from build123d import *

# Parameters (mm, degrees)
F2_R     = 19.05
F3_DEPTH = 55.881
F4_R     = 3.048
F5_R     = 6.35
F6_DEPTH = 19.051


with BuildPart() as f1:
    # F0 (on Front) → F1 (revolve)
    with BuildSketch(Plane.XZ):
        Polygon((0, 55.88), (0, 0), (69.85, 0), (69.85, 19.05), (35.052, 19.05), (35.052, 55.88), align=None)
    revolve(axis=Axis((0, 0, 27.94), (0, 0, -1)))

    # F2 (on face) → F3 (cut, through all)
    with BuildSketch(Plane.XY.offset(55.88)):
        Circle(F2_R)
    extrude(amount=-F3_DEPTH, mode=Mode.SUBTRACT)

    # F4
    f4_edges = [f1.edges().sort_by_distance(p)[0] for p in [
        (-35.052, 0, 55.88),
        (-69.85, 0, 19.05),
        (-35.052, 0, 19.05),
    ]]
    fillet(f4_edges, radius=F4_R)

    # F5 (on face) → F6 (cut, through all)
    with BuildSketch(Plane.XY.offset(19.05)):
        with Locations((-53.848, 0)):
            Circle(F5_R)
        with Locations((0, 53.848)):
            Circle(F5_R)
        with Locations((53.848, 0)):
            Circle(F5_R)
        with Locations((0, -53.848)):
            Circle(F5_R)
    extrude(amount=-F6_DEPTH, mode=Mode.SUBTRACT)


solid = f1.part
Could you check a few things on this model? Use its own coordinates, in mm. A direction names the side the tool comes from. Give positions to 0.01 mm unless a question says otherwise; leave off trailing zeros. Order: outer loops, then holes, each group sorted by start corner. A loop starts at its lowest first (then second) coordinate and runs counter-clockwise, first axis right, second up.
1. I need wall thicknesses on L1, parallel to Y at x = 0, z = 4; L2, parallel to Y at x = 0, z = 24; L3, parallel to X at y = -3.5, z = 15. Which ranges of each line are inside material? Lowest first, please.
2. Suppose I cut it at C-C (z = 25). List the corners of the cut face in (x, y) for me.
3. We'd pull the mould along X, two halves only. Please class faces 3 (the cylindrical face through (33.433, -10.529, 37.68)), 4 (the flat face through (-15, 15, 0)), 5 (the cylindrical face through (-0.827, 60.144, 9.658)), 6 (the cylindrical face through (-0.827, -47.552, 9.658)): pulls with the +X half, pulls with the -X half, needs draft (parallel to the pull), parting line crosses it, or undercut.
4. Will these pins go through, and if not, where does the flat tip stop? P1, Ø7.5, axis at x = 53.848, y = 0, coming from the +Z side; P2, Ø20.5, axis at x = 0, y = -53.848, coming from the +Z side; P3, Ø3, axis at x = 2, z = 29.5, coming from the -Y side; P4, Ø10, axis at x = 26, z = 25, coming from the +Y side (3 decimals).
5. For faces 1 (the cylindrical face through (-60.19, 0.28, 9.66)), 2 (the flat face through (29, 29, 19.05)), which set-ups out of +Z, -Z, +X, -X, +Y, -Y let a thin tool reach every point of the face, with its end or its side?
6. Suppose I cut it at A-A (y = 0). List the corners of the cut face in (x, z) for me.
Solved:
1. L1: y = -69.85 to -60.2, -47.5 to -19.05, 19.05 to 47.5, 60.2 to 69.85
1. L2: y = -35.05 to -19.05, 19.05 to 35.05
1. L3: x = -69.76 to -59.15, -48.55 to -18.73, 18.73 to 48.55, 59.15 to 69.76
2. outline: circle Ø70.1 at (0, 0); hole circle Ø38.1 at (0, 0)
3. face 3: parting line crosses it
3. face 4: needs draft
3. face 5: undercut
3. face 6: undercut
4. P1: passes through
4. P2: stops at z = 19.05
4. P3: stops at y = -35.05
4. P4: stops at y = 28.065
5. face 1: +Z, -Z
5. face 2: +Z
6. outline: (-69.85, 0) - (-60.2, 0) - (-60.2, 19.05) - (-66.8, 19.05) arc R3.05 ccw to (-69.85, 16) - close; (-47.5, 0) - (-19.05, 0) - (-19.05, 55.88) - (-32, 55.88) arc R3.05 ccw to (-35.05, 52.83) - (-35.05, 22.1) arc R3.05 cw to (-38.1, 19.05) - (-47.5, 19.05) - close; (19.05, 0) - (47.5, 0) - (47.5, 19.05) - (38.1, 19.05) arc R3.05 cw to (35.05, 22.1) - (35.05, 52.83) arc R3.05 ccw to (32, 55.88) - (19.05, 55.88) - close; (60.2, 0) - (69.85, 0) - (69.85, 16) arc R3.05 ccw to (66.8, 19.05) - (60.2, 19.05) - close
